For this review, take the finished solid that the model builds, in its own axes (mm). Give positions to 0.01 mm unless a question says otherwise; leave off trailing zeros. Loops run counter-clockwise (first coordinate to the right, second up) from the corner with the lowest first, then second, coordinate; pieces in that order, holes last.
```python
from build123d import *

# Parameters (mm, degrees)
SKETCH1_R           = 28.575
BOSS_EXTRUDE1_DEPTH = 10
SKETCH2_R           = 19.05
CUT_EXTRUDE1_DEPTH  = 42.630052246
SKETCH5_R           = 2.75
CUT_EXTRUDE2_DEPTH  = 65.673434461
SKETCH6_R           = 2.75
CUT_EXTRUDE3_DEPTH  = 42.630052408


with BuildPart() as part:
    # Sketch1 → Boss-Extrude1 (new body)
    with BuildSketch(Plane.XY):
        Circle(SKETCH1_R)
    extrude(amount=BOSS_EXTRUDE1_DEPTH)

    # Sketch2 → Cut-Extrude1 (cut, through all)
    with BuildSketch(Plane.XY.offset(10)):
        Circle(SKETCH2_R)
    extrude(amount=-CUT_EXTRUDE1_DEPTH, mode=Mode.SUBTRACT)

    # Sketch5 → Cut-Extrude2 (cut, through all)
    with BuildSketch(Plane(origin=(0, 28.575, 0), x_dir=(1, 0, 0), z_dir=(0, 1, 0))):
        with Locations(Location((0, -5, 0), (0, 0, 270))):
            Circle(SKETCH5_R)
    extrude(amount=-CUT_EXTRUDE2_DEPTH, mode=Mode.SUBTRACT)

    # Sketch6 → Cut-Extrude3 (cut, through all)
    with BuildSketch(Plane.XY.offset(10)):
        with Locations((-23.8125, 0)):
            Circle(SKETCH6_R)
        with Locations((23.8125, 0)):
            Circle(SKETCH6_R)
    extrude(amount=-CUT_EXTRUDE3_DEPTH, mode=Mode.SUBTRACT)


solid = part.part
```
Item 1: Clearance check with flat-ended pins moving along their axes: pin 1 Ø2 at (y, z) = (5, 1.5) entering from -X; pin 2 Ø4 at (x, z) = (-6, 2) entering from +Y; pin 3 Ø3 at (x, z) = (9, 7.5) entering from +Y. State where each tip first meets the part, or that it passes through.
Answer:
pin 1: stops at x = -28.29
pin 2: stops at y = 28.29
pin 3: stops at y = 27.57
Item 2: For L1, parallel to Z at x = 0, y = 23; L2, parallel to X at y = -25, z = 3.75; L3, parallel to Y at x = 4, z = 5.25, list the stretches that pass through material, from the lowest coordinate up.
Answer:
L1: z = 0 to 2.25, 7.75 to 10
L2: x = -13.84 to -2.45, 2.45 to 13.84
L3: y = -28.29 to -18.63, 18.63 to 28.29
Item 3: Take a section at A-A on x = 0. Give the boundary of the cut face in (y, z) (3 decimals), and give its area (3 significant figures).
Answer:
outline: (-28.575, 0) - (-19.05, 0) - (-19.05, 2.25) - (-28.575, 2.25) - close; (-28.575, 7.75) - (-19.05, 7.75) - (-19.05, 10) - (-28.575, 10) - close; (19.05, 0) - (28.575, 0) - (28.575, 2.25) - (19.05, 2.25) - close; (19.05, 7.75) - (28.575, 7.75) - (28.575, 10) - (19.05, 10) - close
area: 85.7 mm2
Item 4: The part is to be moulded in two halves that separate along Z. For faces 1 (the cylindrical face through (-1.05, -23.65, 7.54)), 2 (the flat face through (19, -6, 10)), 3 (the cylindrical face through (21.065, 0.121, 5.07)), say which applies: released by +Z, released by -Z, zero draft, split by the parting line, or undercut.
Answer:
face 1: undercut
face 2: released by +Z
face 3: zero draft
Item 5: Take a section at D-D on x = 13.5. Give the boundary of the cut face in (y, z).
Answer:
outline: (-25.18, 0) - (-13.44, 0) - (-13.44, 10) - (-25.18, 10) - close; (13.44, 0) - (25.18, 0) - (25.18, 10) - (13.44, 10) - close
Item 6: Take a section at B-B on y = 0. State how many separate pieces and enclosed holes the cut face has, and give its area (3 significant figures).
Answer:
separate pieces: 4
enclosed holes: 0
area: 80.5 mm2
